Autodesk Inventor part; units mm, degrees
ref_plane "YZ Plane" through (0, 0, 0) normal (1, 0, 0) x (0, 1, 0)
ref_plane "XZ Plane" through (0, 0, 0) normal (0, 1, 0) x (-1, 0, 0)
ref_plane "XY Plane" through (0, 0, 0) normal (0, 0, 1) x (1, 0, 0)
sketch "Esquisse1" plane through (0, 0, 0) normal (0, 1, 0) x (-1, 0, 0)
  circle A0 centre (0, 0) radius 5
  dimension "d0" = 10
extrude "Extrusion1" add sketch "Esquisse1" along normal blind 16
sketch "Esquisse2" plane through (0, 16, 0) normal (0, 1, 0) x (1, 0, 0)
  circle A0 centre (0, 0) radius 5
  circle A1 centre (0, 0) radius 2
  dimension "d3" = 4
extrude "Extrusion2" cut sketch "Esquisse2" against normal blind 7 contours A1
thread "Filetage1"
sketch "Esquisse3" plane through (0, 0, 0) normal (0, -1, 0) x (1, 0, 0)
  circle A0 centre (0, 0) radius 5
  circle A1 centre (0, 0) radius 1.6
  dimension "d8" = 3.2
extrude "Extrusion3" cut sketch "Esquisse3" against normal through all contours A1
sketch "Esquisse4" plane through (0, 0, 0) normal (1, 0, 0) x (0, 1, 0)
  circle A0 centre (2, 0) radius 1
  point P0 (0, 0)
  dimension "d11" = 2
extrude "Extrusion4" cut sketch "Esquisse4" along normal through all
thread "Filetage2"
properties part number "Fixation-potar" material "Aluminium 6061"
Geometry: final body of the model. Coordinates: model frame, mm. A direction names the side the tool comes from. Round coordinates to 2 decimals unless told otherwise and drop trailing zeros. Loops run counter-clockwise (first coordinate to the right, second up) from the corner with the lowest first, then second, coordinate; pieces in that order, holes last.
Q1. Section D-D on y = 10.25. Return loops of the section in (x, z), plus the area to 3 significant figures.
Q2. Section C-C on x = 3.5. Return loops of the section in (y, z), plus the area to 3 significant figures.
Q3. Section A-A on x = 0. Return loops of the section in (y, z), plus the area to 3 significant figures.
Q4. Access query for faces 5 (the flat face through (-2.2, 16, 0.1)), 6 (the cylindrical face through (0, 13, 2)). Directions: +Z, -Z, +X, -X, +Y, -Y. A direction counts if a zero-diameter tool reaches every point of the face in a straight line with its end or side. Return the directions, or none.
Q5. Pull-direction query (Z, two-part tool) for faces 1 (the cylindrical face through (-4.77, 7.89, -1.5)), 2 (the flat face through (-2, 0, 0)), 3 (the cylindrical face through (-1.6, 4.44, 0.07)), 4 (the cylindrical face through (3, 3, 0)); classes: released by +Z, released by -Z, zero draft, split by the parting line, or undercut.
Q6. Section B-B on z = 0. Return loops of the section in (x, y).
Q7. Material intervals for L1, parallel to Z at x = 0, y = 4.75; L2, parallel to Y at x = 2.15, z = 0; L3, parallel to Z at x = 0, y = 14.25, sorted ascending.
Q8. Pin query (flat end, axial travel): P1, Ø4.5, axis at x = -0.5, z = -0.5, coming from the +Y side; P2, Ø4, axis at y = 3.5, z = 3, coming from the +X side. Return the tip coordinate at first contact, or that it passes through.
Evaluation:
1. outline: circle Ø10 at (0, 0); hole circle Ø4 at (0, 0)
1. area: 66.0 mm2
2. outline: (0, -3.57) - (16, -3.57) - (16, 3.57) - (0, 3.57) - close; hole circle Ø2 at (2, 0)
2. area: 111 mm2
3. outline: (0, -5) - (16, -5) - (16, -2) - (9, -2) - (9, -1.6) - (0, -1.6) - close; (0, 1.6) - (9, 1.6) - (9, 2) - (16, 2) - (16, 5) - (0, 5) - close
3. area: 103 mm2
4. face 5: +Z, -Z, +X, -X, +Y
4. face 6: +Y
5. face 1: split by the parting line
5. face 2: zero draft
5. face 3: undercut
5. face 4: undercut
6. outline: (-5, 0) - (-1.6, 0) - (-1.6, 9) - (-2, 9) - (-2, 16) - (-5, 16) - close; (1.6, 0) - (5, 0) - (5, 1) - (1.6, 1) - close; (1.6, 3) - (5, 3) - (5, 16) - (2, 16) - (2, 9) - (1.6, 9) - close
7. L1: z = -5 to -1.6, 1.6 to 5
7. L2: y = 0 to 1, 3 to 16
7. L3: z = -5 to -2, 2 to 5
8. P1: stops at y = 16
8. P2: stops at x = 4.9
